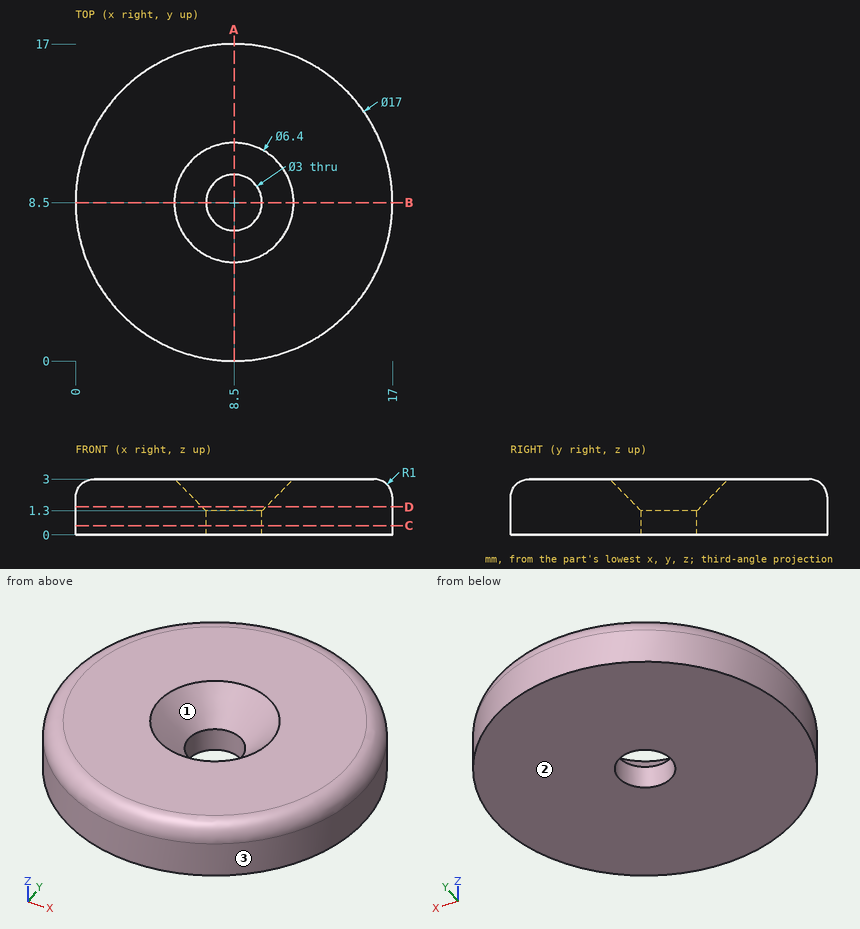
Drawing for the job (mm, zero at the part's lowest x, y, z). Give positions to 0.01 mm unless a question says otherwise; leave off trailing zeros. Loops run counter-clockwise (first coordinate to the right, second up) from the corner with the lowest first, then second, coordinate; pieces in that order, holes last. Notation, with made-up numbers: (51.5, 89) - (71.5, 89) arc R10 cw to (71.5, 104) - close; hole circle Ø9 at (34, 58.5). An arc over 180 degrees is marked (long way). Write item = value, one per line. Start each with the question number.
1) Band-saw the part on C-C on z = 0.5. Give the cut face in (x, y).
2) Band-saw the part on A-A on x = 8.5. Give the cut face in (y, z).
3) Pull direction Y, two halves, no side cores. Call the marked faces 1, 2 and 3: +Y half, -Y half, draft (parallel to the pull), parting line (faces both ways), or undercut.
4) Probe probe 1 along Y at (x, z) = (8.5, 0.5); probe 2 along X at (y, z) = (8, 2.1) (3 decimals); probe 3 along X at (y, z) = (7.75, 1.55). List the from-to ranges inside material, lowest first. Write a range as from..to.
5) Drop a flat-ended pin along its axis: pin 1 Ø5 at (x, y) = (8.5, 8.5) entering from +Z. Give the stop position or say it passes through.
6) Band-saw the part on D-D on z = 1.5. Give the cut face in (x, y), plus the area to 3 significant figures.
Final values:
q1.outline = circle Ø17 at (8.5, 8.5); hole circle Ø3 at (8.5, 8.5)
q2.outline = (0, 0) - (7, 0) - (7, 1.3) - (5.3, 3) - (1, 3) arc R1 ccw to (0, 2) - close; (10, 0) - (17, 0) - (17, 2) arc R1 ccw to (16, 3) - (11.7, 3) - (10, 1.3) - close
q3.face_1 = undercut
q3.face_2 = draft
q3.face_3 = parting line
q4.probe_1 = 0..7, 10..17
q4.probe_2 = 0.02..6.255, 10.745..16.98
q4.probe_3 = 0.03..6.92, 10.08..16.97
q5.pin_1 = 2.3
q6.outline = circle Ø17 at (8.5, 8.5); hole circle Ø3.4 at (8.5, 8.5)
q6.area = 218 mm²
